Verification items for the finished model (mm, model axes). Coordinates: 2 decimals unless noted, no trailing zeros. Order: outer loops, then holes, each group sorted by start corner. A loop starts at its lowest first (then second) coordinate and runs counter-clockwise, first axis right, second up. Notation, with made-up numbers: M 47,69 L 84,69 A27 ccw 84,97 Z; hole C -7,-19.75 d10. An arc over 180 degrees is marked long. Return JSON: item names as keys, results as strings. Group by question number.
1. Section check D-D, the plane y = 5.75. Record the cut outline in (x, z), plus the area to 3 significant figures.
2. Mould release check, pull along X, two halves, no side actions. Record for faces 1 (the cylindrical face through (1.27, 8.61, -0.4)), 2 (the cylindrical face through (-6, 5, 0)), 3 (the flat face through (1.2, 9.6, 1.2)): +X half, -X half, draft (parallel to the pull), parting line (faces both ways), or undercut.
3. Material ranges on line 1 along X through (y, z) = (8.8, 0); line 2 along X through (y, z) = (7.4, 0); line 3 along Y through (x, z) = (-3.5, 3.5), recorded low to high.
4. Section check A-A, the plane z = 0. Record the cut outline in (x, y).
5. Gauge pin test, flat ends, axial feed: pin 1 (3 mm diameter, centred on x = 2.5, z = -1, fed in from -Y); pin 2 (4 mm diameter, centred on x = 1, z = -0.5, fed in from -Y); pin 3 (3 mm diameter, centred on y = 5.5, z = -2, fed in from +X); pin 4 (1.6 mm diameter, centred on x = 0, z = 0, fed in from +Y). Record the tip position at first contact, or that the pin passes through.
6. Section check C-C, the plane x = 3.75. Record the cut outline in (y, z), plus the area to 3 significant figures.
7. Section check B-B, the plane x = 0. Record the cut outline in (y, z).
```python
from build123d import *

# Parameters (mm, degrees)
SKETCH1_R           = 6
BOSS_EXTRUDE1_DEPTH = 9.6
SKETCH2_R           = 1.33
CUT_EXTRUDE1_DEPTH  = 3
SKETCH3_R           = 5
CUT_EXTRUDE2_DEPTH  = 1
SKETCH4_R           = 0.3
BOSS_EXTRUDE2_DEPTH = 1


with BuildPart() as part:
    # Sketch1 → Boss-Extrude1 (new body)
    with BuildSketch(Plane(origin=(0, 0, 0), x_dir=(1, 0, 0), z_dir=(0, 1, 0))):
        Circle(SKETCH1_R)
    extrude(amount=BOSS_EXTRUDE1_DEPTH)

    # Sketch2 → Cut-Extrude1 (cut)
    with BuildSketch(Plane(origin=(0, 9.6, 0), x_dir=(1, 0, 0), z_dir=(0, 1, 0))):
        Circle(SKETCH2_R)
    extrude(amount=-CUT_EXTRUDE1_DEPTH, mode=Mode.SUBTRACT)

    # Sketch3 → Cut-Extrude2 (cut)
    with BuildSketch(Plane(origin=(0, 6.6, 0), x_dir=(1, 0, 0), z_dir=(0, 1, 0))):
        Circle(SKETCH3_R)
    extrude(amount=CUT_EXTRUDE2_DEPTH, mode=Mode.SUBTRACT)

    # Sketch4 → Boss-Extrude2 (add)
    with BuildSketch(Plane.XZ):
        with Locations((-3.75, 0)):
            Circle(SKETCH4_R)
        with Locations((3.75, 0)):
            Circle(SKETCH4_R)
    extrude(amount=BOSS_EXTRUDE2_DEPTH)


solid = part.part
```
Answers follow:
{
 "1": {"outline": "C 0,0 d12", "area": "113 mm^2"},
 "2": {"face 1": "undercut", "face 2": "parting line", "face 3": "draft"},
 "3": {"line 1": "-6 to -1.33, 1.33 to 6", "line 2": "-6 to -5, 5 to 6", "line 3": "0 to 6.6, 7.6 to 9.6"},
 "4": {"outline": "M -6,0 L -4.05,0 L -4.05,-1 L -3.45,-1 L -3.45,0 L 3.45,0 L 3.45,-1 L 4.05,-1 L 4.05,0 L 6,0 L 6,9.6 L 1.33,9.6 L 1.33,7.6 L 5,7.6 L 5,6.6 L -5,6.6 L -5,7.6 L -1.33,7.6 L -1.33,9.6 L -6,9.6 Z"},
 "5": {"pin 1": "y = -1", "pin 2": "y = 0", "pin 3": "x = 5.98", "pin 4": "y = 6.6"},
 "6": {"outline": "M -1,-0.3 L 0,-0.3 L 0,-4.68 L 9.6,-4.68 L 9.6,4.68 L 0,4.68 L 0,0.3 L -1,0.3 Z; hole M 6.6,-3.31 L 7.6,-3.31 L 7.6,3.31 L 6.6,3.31 Z", "area": "83.9 mm^2"},
 "7": {"outline": "M 0,-6 L 9.6,-6 L 9.6,-1.33 L 7.6,-1.33 L 7.6,-5 L 6.6,-5 L 6.6,5 L 7.6,5 L 7.6,1.33 L 9.6,1.33 L 9.6,6 L 0,6 Z"}
}
